from build123d import *

# Parameters (mm, degrees)
F0_W     = 86
F0_H     = 57
F1_DEPTH = 3
F2_W     = 78.7
F2_H     = 55.2
F3_DEPTH = 3
F4_R     = 1.5
F5_DEPTH = 25
F6_W     = 33.5
F6_H     = 5
F7_DEPTH = 13.73


with BuildPart() as f1:
    # F0 (on Top) → F1 (new body)
    with BuildSketch(Plane.XY):
        Rectangle(F0_W, F0_H)
    extrude(amount=F1_DEPTH)

    # F2 (on face) → F3 (join)
    with BuildSketch(Plane.XY.offset(3)):
        with Locations((3.65, -0.9)):
            Rectangle(F2_W, F2_H)
    extrude(amount=F3_DEPTH)

    # F4 (on face) → F5 (cut)
    with BuildSketch(Plane.XY.offset(3)):
        with Locations((-40.812388, 26.41947)):
            Circle(F4_R)
        with Locations((-40.812388, 22.852236)):
            Circle(F4_R)
    extrude(amount=-F5_DEPTH, mode=Mode.SUBTRACT)

    # F6 (on face) → F7 (join)
    with BuildSketch(Plane(origin=(0, 0, 0), x_dir=(1, 0, 0), z_dir=(0, 0, -1))):
        with Locations((26.25, 26)):
            Rectangle(F6_W, F6_H)
    extrude(amount=F7_DEPTH)


solid = f1.part
Geometry: final body of the model. Coordinates: model frame, mm. A direction names the side the tool comes from. Coordinates: 2 decimals unless noted, no trailing zeros. Order: outer loops, then holes, each group sorted by start corner. A loop starts at its lowest first (then second) coordinate and runs counter-clockwise, first axis right, second up. Notation, with made-up numbers: (-26, 69) - (-8, 69) arc R32 cw to (-8, 100) - close; hole circle Ø10 at (13.5, 85). An arc over 180 degrees is marked (long way). Use one line per item in the form item = value.
1) Pin query (flat end, axial travel): pin 1 (5 mm diameter, centred on x = -40.81, y = 22.85, fed in from +Z); pin 2 (10 mm diameter, centred on x = 7.5, y = -2, fed in from -Z); pin 3 (1.5 mm diameter, centred on x = 3.5, z = 4, fed in from +Y). Return the tip coordinate at first contact, or that it passes through.
Solutions:
pin_1 = 3
pin_2 = 0
pin_3 = 26.7
2) Section B-B (y = 9). Return loops of the section in (x, z), then the cut area to 3 significant figures.
Solutions:
outline = (-43, 0) - (43, 0) - (43, 6) - (-35.7, 6) - (-35.7, 3) - (-43, 3) - close
area = 494 mm^2
3) Section C-C (z = 4). Return loops of the section in (x, y), then the cut area to 3 significant figures.
Solutions:
outline = (-35.7, -28.5) - (43, -28.5) - (43, 26.7) - (-35.7, 26.7) - close
area = 4,340 mm^2
4) Section A-A (x = 11). Return loops of the section in (y, z), then the cut area to 3 significant figures.
Solutions:
outline = (-28.5, -13.73) - (-23.5, -13.73) - (-23.5, 0) - (28.5, 0) - (28.5, 3) - (26.7, 3) - (26.7, 6) - (-28.5, 6) - close
area = 405 mm^2
5) Ray query, L1, parallel to Y at x = 37.5, z = -11; L2, parallel to X at y = 22, z = 4; L3, parallel to Z at x = -21, y = -21. Return the intervals inside material, ascending.
Solutions:
L1 = -28.5 to -23.5
L2 = -35.7 to 43
L3 = 0 to 6
6) Section D-D (x = -33.5). Return loops of the section in (y, z).
Solutions:
outline = (-28.5, 0) - (28.5, 0) - (28.5, 3) - (26.7, 3) - (26.7, 6) - (-28.5, 6) - close
7) Set-up query: faces 1 (the face through (-35.7, -1, 4)), 2 (the face through (3, 26.7, 4)), 3 (the face through (26, -23.5, -7)), 4 (the face through (-43, 0, 1)), 5 (the face through (9.5, -26, -7)). Return all of +Z, -Z, +X, -X, +Y, -Y with unobstructed straight access to the full face (end or side cutting, diameter ignored); none if empty.
Solutions:
face_1 = +Z, -X, +Y, -Y
face_2 = +Z, +X, -X, +Y
face_3 = -Z, +X, -X, +Y
face_4 = +Z, -Z, -X, +Y, -Y
face_5 = -Z, -X, +Y, -Y
